from build123d import *

# Parameters (mm, degrees)
F0_R     = 22.5
F1_DEPTH = 3
F2_R     = 10
F3_DEPTH = 70
F4_R     = 24
F5_DEPTH = 28


with BuildPart() as f1:
    # F0 (on Top) → F1 (new body)
    with BuildSketch(Plane.XY):
        Circle(F0_R)
    extrude(amount=F1_DEPTH)

    # F2 (on Top) → F3 (join)
    with BuildSketch(Plane.XY):
        Circle(F2_R)
    extrude(amount=F3_DEPTH)

    # F4 (on face) → F5 (join)
    with BuildSketch(Plane(origin=(0, 0, 0), x_dir=(1, 0, 0), z_dir=(0, 0, -1))):
        Circle(F4_R)
    extrude(amount=F5_DEPTH)


solid = f1.part
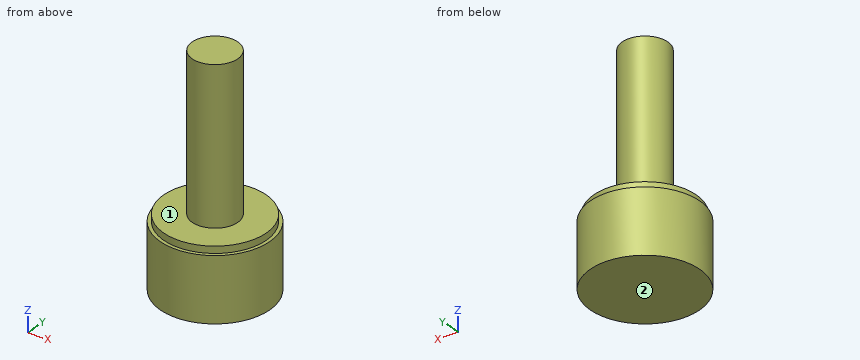
Build history of the part. All positions in model axes, mm. Face numbers are marked on the shaded views. A direction names the side the tool comes from. Coordinates: 2 decimals unless noted, no trailing zeros. Order: outer loops, then holes, each group sorted by start corner. A loop starts at its lowest first (then second) coordinate and runs counter-clockwise, first axis right, second up. Notation, with made-up numbers: (78, 6) - (112, 6) arc R26 cw to (112, 26) - close; hole circle Ø5 at (69, 65.25). An arc over 180 degrees is marked (long way). Put each result on its own line as item: value.
1. Saw through at C-C (y = 5). Write the cut outline in (x, z).
Answer sheet:
outline: (-23.47, -28) - (23.47, -28) - (23.47, 0) - (21.94, 0) - (21.94, 3) - (8.66, 3) - (8.66, 70) - (-8.66, 70) - (-8.66, 3) - (-21.94, 3) - (-21.94, 0) - (-23.47, 0) - close
2. Probe line 1 along Z through (x, y) = (12, 7.5); line 2 along Y through (x, z) = (-0.5, 27); line 3 along Z through (x, y) = (8.5, 21). List the from-to ranges inside material, lowest first. Write a range as [from, to].
Answer sheet:
line 1: z = [-28, 3]
line 2: y = [-9.99, 9.99]
line 3: z = [-28, 0]
3. Saw through at B-B (z = 41). Write the cut outline in (x, y), and give its area (3 significant figures).
Answer sheet:
outline: circle Ø20 at (0, 0)
area: 314 mm^2
4. Saw through at A-A (x = 0). Write the cut outline in (y, z), and give its area (3 significant figures).
Answer sheet:
outline: (-24, -28) - (24, -28) - (24, 0) - (22.5, 0) - (22.5, 3) - (10, 3) - (10, 70) - (-10, 70) - (-10, 3) - (-22.5, 3) - (-22.5, 0) - (-24, 0) - close
area: 2,820 mm^2
5. Saw through at D-D (x = -11.5). Write the cut outline in (y, z), and give its area (3 significant figures).
Answer sheet:
outline: (-21.07, -28) - (21.07, -28) - (21.07, 0) - (19.34, 0) - (19.34, 3) - (-19.34, 3) - (-19.34, 0) - (-21.07, 0) - close
area: 1,300 mm^2
6. Tool access for the marked faces 1 and 2: list every direction of +Z, -Z, +X, -X, +Y, -Y with a clear straight run to the whole face (end or side of a thin tool).
Answer sheet:
face 1: +Z
face 2: -Z, +X, -X, +Y, -Y
7. Drop flat-ended pins along their axis: P1, Ø1.5, axis at x = 5.5, y = 18.5, coming from the +Z side; P2, Ø2, axis at x = -6, z = 14.5, coming from the +Y side; P3, Ø1, axis at x = -11, z = -9.5, coming from the -Y side. Give the stop position or say it passes through.
Answer sheet:
P1: stops at z = 3
P2: stops at y = 8.66
P3: stops at y = -21.58
